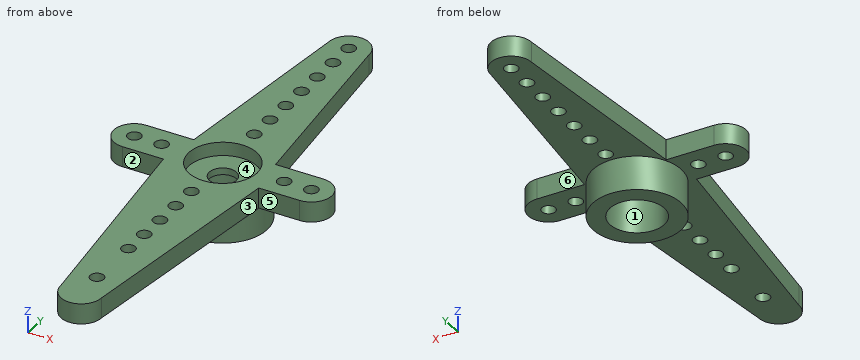
from build123d import *

# Parameters (mm, degrees)
SKETCH_1_R          = 0.5
SKETCH_1_R_2        = 1
EXTRUDE_1_DEPTH     = 1.5
SKETCH_2_R          = 3.25
SKETCH_2_R_2        = 2
EXTRUDE_2_DEPTH     = 2.5
SKETCH_3_R          = 2.5
CUT_EXTRUDE_1_DEPTH = 1


with BuildPart() as part:
    # 草图1 → 凸台-拉伸1 (new body)
    with BuildSketch(Plane.XY):
        with BuildLine():
            Line((1.5, 16), (3, 1.5))
            Line((3, 1.5), (6.5, 1.5))
            ThreePointArc((6.5, 1.5), (8, 0), (6.5, -1.5))
            Line((6.5, -1.5), (3.5, -1.5))
            Line((3.5, -1.5), (1.5, -18))
            ThreePointArc((1.5, -18), (0, -19.5), (-1.5, -18))
            Line((-1.5, -18), (-3.5, -1.5))
            Line((-3.5, -1.5), (-6.5, -1.5))
            ThreePointArc((-6.5, -1.5), (-8, 0), (-6.5, 1.5))
            Line((-6.5, 1.5), (-3, 1.5))
            Line((-3, 1.5), (-1.5, 16))
            ThreePointArc((-1.5, 16), (0, 17.5), (1.5, 16))
        make_face()
        with Locations((-6.5, 0)):
            Circle(SKETCH_1_R, mode=Mode.SUBTRACT)
        Circle(SKETCH_1_R_2, mode=Mode.SUBTRACT)
        with Locations((-4.5, 0)):
            Circle(SKETCH_1_R, mode=Mode.SUBTRACT)
        with Locations(Location((4.5, 0, 0), (0, 0, 180))):
            Circle(SKETCH_1_R, mode=Mode.SUBTRACT)
        with Locations(Location((6.5, 0, 0), (0, 0, 180))):
            Circle(SKETCH_1_R, mode=Mode.SUBTRACT)
        with Locations((0, 16)):
            Circle(SKETCH_1_R, mode=Mode.SUBTRACT)
        with Locations((0, 14)):
            Circle(SKETCH_1_R, mode=Mode.SUBTRACT)
        with Locations((0, 12)):
            Circle(SKETCH_1_R, mode=Mode.SUBTRACT)
        with Locations((0, 10)):
            Circle(SKETCH_1_R, mode=Mode.SUBTRACT)
        with Locations((0, 8)):
            Circle(SKETCH_1_R, mode=Mode.SUBTRACT)
        with Locations((0, 6)):
            Circle(SKETCH_1_R, mode=Mode.SUBTRACT)
        with Locations((0, 4)):
            Circle(SKETCH_1_R, mode=Mode.SUBTRACT)
        with Locations(Location((0, -16, 0), (0, 0, 180))):
            Circle(SKETCH_1_R, mode=Mode.SUBTRACT)
        with Locations(Location((0, -4, 0), (0, 0, 180))):
            Circle(SKETCH_1_R, mode=Mode.SUBTRACT)
        with Locations(Location((0, -6, 0), (0, 0, 180))):
            Circle(SKETCH_1_R, mode=Mode.SUBTRACT)
        with Locations(Location((0, -8, 0), (0, 0, 180))):
            Circle(SKETCH_1_R, mode=Mode.SUBTRACT)
        with Locations(Location((0, -10, 0), (0, 0, 180))):
            Circle(SKETCH_1_R, mode=Mode.SUBTRACT)
        with Locations(Location((0, -12, 0), (0, 0, 180))):
            Circle(SKETCH_1_R, mode=Mode.SUBTRACT)
    extrude(amount=EXTRUDE_1_DEPTH)

    # 草图2 → 凸台-拉伸2 (add)
    with BuildSketch(Plane(origin=(0, 0, 0), x_dir=(-1, 0, 0), z_dir=(0, 0, -1))):
        with Locations(Location((0, 0, 0), (0, 0, 180))):
            Circle(SKETCH_2_R)
        Circle(SKETCH_2_R_2, mode=Mode.SUBTRACT)
    extrude(amount=EXTRUDE_2_DEPTH)

    # 草图3 → 切除-拉伸1 (cut)
    with BuildSketch(Plane.XY.offset(1.5)):
        Circle(SKETCH_3_R)
    extrude(amount=-CUT_EXTRUDE_1_DEPTH, mode=Mode.SUBTRACT)


solid = part.part
Geometry: final body of the model. Coordinates: model frame, mm. Face numbers are marked on the shaded views. A direction names the side the tool comes from. Give positions to 0.01 mm unless a question says otherwise; leave off trailing zeros. Order: outer loops, then holes, each group sorted by start corner. A loop starts at its lowest first (then second) coordinate and runs counter-clockwise, first axis right, second up. Notation, with made-up numbers: (-33.5, 13.25) -> (-29.5, 13.25) arc R18 cw to (-29.5, 45.25) -> close; hole circle Ø3 at (39, -29.75). An arc over 180 degrees is marked (long way). Answer as a JSON object with one key per item and string values.
Q1. Section B-B (x = 0). State how many separate pieces and enclosed holes the cut face has, plus the area to 4 significant figures.
Entries:
{"separate pieces": "15", "enclosed holes": "0", "area": "36.25 mm^2"}
Q2. Material intervals for probe 1 along Y at (x, z) = (0.75, -1.4); probe 2 along Z at (x, y) = (-0.5, 13); probe 3 along Y at (x, z) = (-5.25, 0.25), sorted ascending.
Entries:
{"probe 1": "y = -3.16 to -1.85, 1.85 to 3.16", "probe 2": "z = 0 to 1.5", "probe 3": "y = -1.5 to 1.5"}
Q3. Draft query along X for the marked faces 1, 2 and 3. Return one class per face: released by +X, released by -X, zero draft, split by the parting line, or undercut.
Entries:
{"face 1": "undercut", "face 2": "zero draft", "face 3": "released by +X"}
Q4. Section D-D (y = -4). Output: boundary loops of the cut face in (x, z).
Entries:
{"outline": "(-3.2, 0) -> (-0.5, 0) -> (-0.5, 1.5) -> (-3.2, 1.5) -> close; (0.5, 0) -> (3.2, 0) -> (3.2, 1.5) -> (0.5, 1.5) -> close"}
Q5. Section C-C (z = -1.4). Output: boundary loops of the cut face in (x, y), plus the area to 3 significant figures.
Entries:
{"outline": "circle Ø6.5 at (0, 0); hole circle Ø4 at (0, 0)", "area": "20.6 mm^2"}
Q6. First-contact query: pin 1 (1.2 mm diameter, centred on x = 0, y = 0, fed in from -Z); pin 2 (8 mm diameter, centred on x = 2.5, y = 7, fed in from -Z); pin 3 (1.5 mm diameter, centred on x = 2, z = 0.5, fed in from -Y); pin 4 (2.5 mm diameter, centred on x = -1, y = 0, fed in from +Z). Flat tips, straight axial feed; report the tip coordinate or a pass-through.
Entries:
{"pin 1": "passes through", "pin 2": "stops at z = 0", "pin 3": "stops at y = -18.83", "pin 4": "stops at z = 0.5"}
Q7. Access query for the marked faces 4, 5 and 6. Directions: +Z, -Z, +X, -X, +Y, -Y. A direction counts if a zero-diameter tool reaches every point of the face in a straight line with its end or side. Return the directions, or none.
Entries:
{"face 4": "+Z", "face 5": "+Z, -Z, +X, -Y", "face 6": "+Z, -Z, +X, +Y"}
Q8. Section A-A (y = 6). Output: boundary loops of the cut face in (x, z).
Entries:
{"outline": "(-2.53, 0) -> (-0.5, 0) -> (-0.5, 1.5) -> (-2.53, 1.5) -> close; (0.5, 0) -> (2.53, 0) -> (2.53, 1.5) -> (0.5, 1.5) -> close"}
